Geometry: final body of the model. Coordinates: model frame, mm. Face numbers are marked on the shaded views. A direction names the side the tool comes from. Coordinates: 2 decimals unless noted, no trailing zeros. Order: outer loops, then holes, each group sorted by start corner. A loop starts at its lowest first (then second) coordinate and runs counter-clockwise, first axis right, second up. Notation, with made-up numbers: M 56,-0.75 L 94,-0.75 A13 cw 94,18.25 Z; hole C 23,84.5 d11. An arc over 180 degrees is marked long. One line per question, with ' | ' between items.
from build123d import *

# Parameters (mm, degrees)
F1_DEPTH = 30
F2_R     = 4.4
F3_R     = 4.4
F4_DEPTH = 25


# Not quite as in the source:
# - a feature names something its author has since deleted; it is built from what else it names


with BuildPart() as f1:
    # F0 (on Front) → F1 (new body)
    with BuildSketch(Plane.XZ):
        Polygon((90, -1), (90, 1), (70, 1), (70, 79), (-70, 79), (-70, 1), (-90, 1), (-90, -1), (-68, -1), (-68, 77), (68, 77), (68, -1), align=None)
    extrude(amount=F1_DEPTH)

    # F2 (on face) + F3 (on face) → F4 (cut)
    with BuildSketch(Plane.XY.offset(1)):
        with Locations((-80, -15)):
            Circle(F2_R)
        with Locations((80, -15)):
            Circle(F2_R)
    with BuildSketch(Plane.XY.offset(79)):
        with Locations((-37.5, -15)):
            Circle(F3_R)
        with Locations((37.5, -15)):
            Circle(F3_R)
    extrude(amount=-F4_DEPTH, mode=Mode.SUBTRACT)


solid = f1.part
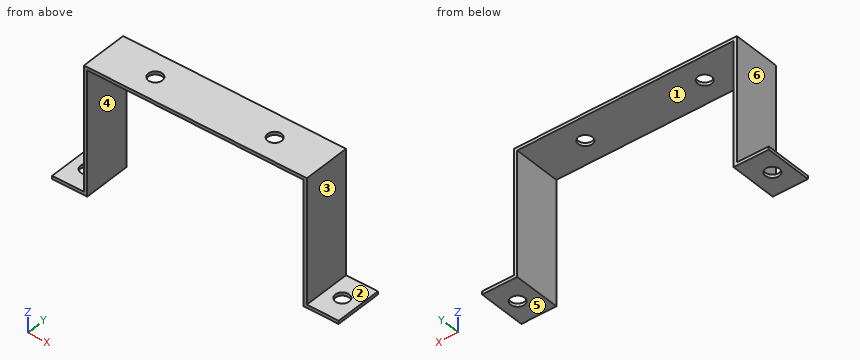
1. Pin query (flat end, axial travel): P1, Ø9, axis at y = -14, z = 24, coming from the -X side; P2, Ø6, axis at x = -82.5, y = -22, coming from the +Z side; P3, Ø2, axis at x = -15.5, y = -4.5, coming from the -Z side. Return the tip coordinate at first contact, or that it passes through.
Response values:
P1: stops at x = -70 | P2: stops at z = 1 | P3: stops at z = 77
2. Section D-D, the plane x = -15. Output: boundary loops of the cut face in (y, z).
Response values:
outline: M -30,77 L 0,77 L 0,79 L -30,79 Z
3. Access query for the marked faces 4, 5 and 6. Directions: +Z, -Z, +X, -X, +Y, -Y. A direction counts if a zero-diameter tool reaches every point of the face in a straight line with its end or side. Return the directions, or none.
Response values:
face 4: -Z, +Y, -Y | face 5: -Z, +X, -X, +Y, -Y | face 6: +Z, -X, +Y, -Y
4. Section A-A, the plane y = -15. Output: boundary loops of the cut face in (x, z).
Response values:
outline: M -90,-1 L -84.4,-1 L -84.4,1 L -90,1 Z; M -75.6,-1 L -68,-1 L -68,77 L -41.9,77 L -41.9,79 L -70,79 L -70,1 L -75.6,1 Z; M -33.1,77 L 33.1,77 L 33.1,79 L -33.1,79 Z; M 41.9,77 L 68,77 L 68,-1 L 75.6,-1 L 75.6,1 L 70,1 L 70,79 L 41.9,79 Z; M 84.4,-1 L 90,-1 L 90,1 L 84.4,1 Z
5. Section B-B, the plane x = -37.5. Output: boundary loops of the cut face in (y, z), and give its area (3 significant figures).
Response values:
outline: M -30,77 L -19.4,77 L -19.4,79 L -30,79 Z; M -10.6,77 L 0,77 L 0,79 L -10.6,79 Z | area: 42.4 mm^2
6. Draft query along X for the marked faces 1, 2 and 3. Return one class per face: pulls with the +X half, pulls with the -X half, needs draft (parallel to the pull), parting line crosses it, or undercut.
Response values:
face 1: undercut | face 2: needs draft | face 3: pulls with the +X half
7. Section C-C, the plane z = 37.5. Output: boundary loops of the cut face in (x, y), and give its area (3 significant figures).
Response values:
outline: M -70,-30 L -68,-30 L -68,0 L -70,0 Z; M 68,-30 L 70,-30 L 70,0 L 68,0 Z | area: 120 mm^2
8. Material intervals for line 1 (Y direction, x = 37.5, z = 77.8); line 2 (X direction, y = -24.75, z = 39.5); line 3 (Z direction, x = -71, y = -8.75), sorted ascending. Write a range as [from, to].
Response values:
line 1: y = [-30, -19.4], [-10.6, 0] | line 2: x = [-70, -68], [68, 70] | line 3: z = [-1, 1]
